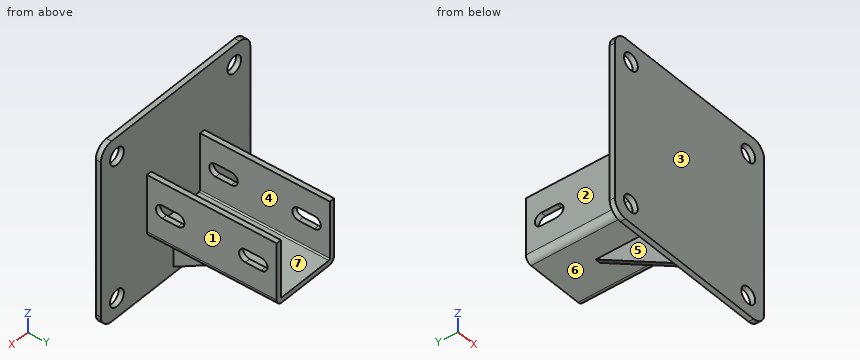
```python
from build123d import *

# Parameters (mm, degrees)
SKETCH_2_W          = 140
SKETCH_2_H          = 140
EXTRUDE_1_DEPTH     = 4
EXTRUDE_1_2_DEPTH   = 100
EXTRUDE_2_DEPTH     = 2
CUT_EXTRUDE_1_DEPTH = 98
SKETCH_6_R          = 6.5
CUT_EXTRUDE_2_DEPTH = 5
FILLET_1_R          = 10


with BuildPart() as part:
    # Эскиз2 → Extrude 1 (new body)
    with BuildSketch(Plane(origin=(0, 0, 0), x_dir=(1, 0, 0), z_dir=(0, 1, 0))):
        Rectangle(SKETCH_2_W, SKETCH_2_H)
    extrude(amount=EXTRUDE_1_DEPTH)

    # Эскиз3 → Extrude 1 2 (add)
    with BuildSketch(Plane(origin=(0, 4, 0), x_dir=(1, 0, 0), z_dir=(0, 1, 0))):
        with BuildLine():
            Line((-23, -22.5), (-23, 21.5))
            ThreePointArc((-23, 21.5), (-22.707106781, 22.207106781), (-22, 22.5))
            Line((-22, 22.5), (22, 22.5))
            ThreePointArc((22, 22.5), (22.707106781, 22.207106781), (23, 21.5))
            Line((23, 21.5), (23, -22.5))
            Line((23, -22.5), (27, -22.5))
            Line((27, -22.5), (27, 21.5))
            ThreePointArc((27, 21.5), (25.535533906, 25.035533906), (22, 26.5))
            Line((22, 26.5), (-22, 26.5))
            ThreePointArc((-22, 26.5), (-25.535533906, 25.035533906), (-27, 21.5))
            Line((-27, 21.5), (-27, -22.5))
            Line((-27, -22.5), (-23, -22.5))
        make_face()
    extrude(amount=EXTRUDE_1_2_DEPTH)

    # Эскиз4 → Бобышка-Вытянуть2 (add, symmetric)
    with BuildSketch(Plane(origin=(0, 0, 0), x_dir=(0, 0, -1), z_dir=(1, 0, 0))):
        Polygon((26.5, 70.683956091), (65, 4), (26.5, 4), align=None)
    extrude(amount=EXTRUDE_2_DEPTH, both=True)

    # Эскиз5 → Вырез-Вытянуть1 (cut, through all)
    with BuildSketch(Plane(origin=(27, 0, 0), x_dir=(0, 0, -1), z_dir=(1, 0, 0))):
        with BuildLine():
            Line((5, 92), (5, 80))
            ThreePointArc((5, 80), (0, 75), (-5, 80))
            Line((-5, 80), (-5, 92))
            ThreePointArc((-5, 92), (0, 97), (5, 92))
        make_face()
        with BuildLine():
            Line((5, 28), (5, 16))
            ThreePointArc((5, 16), (0, 11), (-5, 16))
            Line((-5, 16), (-5, 28))
            ThreePointArc((-5, 28), (0, 33), (5, 28))
        make_face()
    extrude(amount=-CUT_EXTRUDE_1_DEPTH, mode=Mode.SUBTRACT)

    # Эскиз6 → Вырез-Вытянуть2 (cut, through all)
    with BuildSketch(Plane(origin=(0, 4, 0), x_dir=(1, 0, 0), z_dir=(0, 1, 0))):
        with Locations(Location((-55, 55, 0), (0, 0, 270))):  # turned: the seam where the file's is
            Circle(SKETCH_6_R)
        with Locations(Location((-55, -55, 0), (0, 0, 270))):  # turned: the seam where the file's is
            Circle(SKETCH_6_R)
        with Locations(Location((55, 55, 0), (0, 0, 270))):  # turned: the seam where the file's is
            Circle(SKETCH_6_R)
        with Locations(Location((55, -55, 0), (0, 0, 270))):  # turned: the seam where the file's is
            Circle(SKETCH_6_R)
    extrude(amount=-CUT_EXTRUDE_2_DEPTH, mode=Mode.SUBTRACT)

    # Скругление1
    fillet_1_edges = [part.edges().sort_by_distance(p)[0] for p in [
        (70, 2, 70),
        (-70, 2, 70),
        (-70, 2, -70),
        (70, 2, -70),
    ]]
    fillet(fillet_1_edges, radius=FILLET_1_R)


solid = part.part
```
The model under review builds one solid part; all positions refer to its coordinate system, in mm. Face numbers are marked on the shaded views. A direction names the side the tool comes from. Round coordinates to 2 decimals unless told otherwise and drop trailing zeros. Write each loop counter-clockwise with the first axis right and the second up, starting at its lowest first coordinate (ties: lowest second). Pieces come first, ordered by that corner, then holes. Notation, with made-up numbers: M 64.25,7.25 L 115.25,7.25 A26 ccw 115.25,22.25 Z; hole C 79.5,-26.5 d3. An arc over 180 degrees is marked long. Use CSV: the item, a comma, the result in double quotes. Start each with the question number.
(1) We need section D-D, the plane z = 55. State the section outline as (x, y) points.
(2) We need section B-B, the plane y = 95. State the section outline as (x, z) points.
(3) Tool access review of the marked faces 1, 2 and 3: name each direction out of +Z, -Z, +X, -X, +Y, -Y from which nothing blocks a thin tool from reaching the whole face with its end or side.
(4) We need section C-C, the plane z = 0. State the section outline as (x, y) points, then the cut area to 3 significant figures.
(5) For line 1 along X through (y, z) = (2, 55); line 2 along X through (y, z) = (18, -8.5); line 3 along Y through (x, z) = (-20, 54), list the stretches that pass through material, from the lowest coordinate up.
(6) The part is to be moulded in two halves that separate along X. For the marked faces 4, 5, 6 and 7, say which applies: +X half, -X half, draft (parallel to the pull), parting line (faces both ways), or undercut.
(7) We need section A-A, the plane x = 52.5. State the section outline as (y, z) points.
(8) Clearance check with flat-ended pins moving along their axes: P1, Ø2, axis at x = -25, y = 88.5, coming from the -Z side; P2, Ø1.2, axis at x = -25, y = 89, coming from the +Z side; P3, Ø8, axis at y = 44, z = 21, coming from the -X side; P4, Ø8, axis at x = -55, z = -55, coming from the -Y side. State where each tip first meets the part, or that it passes through.
Findings:
1,outline,"M -70,0 L -61.5,0 L -61.5,4 L -70,4 Z; M -48.5,0 L 48.5,0 L 48.5,4 L -48.5,4 Z; M 61.5,0 L 70,0 L 70,4 L 61.5,4 Z"
2,outline,"M -27,-21.5 A5 ccw -22,-26.5 L 22,-26.5 A5 ccw 27,-21.5 L 27,-4 L 23,-4 L 23,-21.5 A1 cw 22,-22.5 L -22,-22.5 A1 cw -23,-21.5 L -23,-4 L -27,-4 Z; M -27,4 L -23,4 L -23,22.5 L -27,22.5 Z; M 23,4 L 27,4 L 27,22.5 L 23,22.5 Z"
3,face 1,"+Z, -Z, +X, +Y"
3,face 2,"+Z, -Z, -X, +Y"
3,face 3,"+Z, -Z, +X, -X, -Y"
4,outline,"M -70,0 L 70,0 L 70,4 L 27,4 L 27,11 L 23,11 L 23,4 L -23,4 L -23,11 L -27,11 L -27,4 L -70,4 Z; M -27,33 L -23,33 L -23,75 L -27,75 Z; M -27,97 L -23,97 L -23,104 L -27,104 Z; M 23,33 L 27,33 L 27,75 L 23,75 Z; M 23,97 L 27,97 L 27,104 L 23,104 Z"
4,area,"1,010 mm^2"
5,line 1,"-70 to -61.5, -48.5 to 48.5, 61.5 to 70"
5,line 2,"-27 to -23, 23 to 27"
5,line 3,"0 to 4"
6,face 4,"undercut"
6,face 5,"-X half"
6,face 6,"draft"
6,face 7,"undercut"
7,outline,"M 0,-70 L 4,-70 L 4,-61 L 0,-61 Z; M 0,-49 L 4,-49 L 4,49 L 0,49 Z; M 0,61 L 4,61 L 4,70 L 0,70 Z"
8,P1,"z = -26.08"
8,P2,"z = 22.5"
8,P3,"x = -27"
8,P4,"through"
